For this review, take the finished solid that the model builds, in its own axes (mm). A direction names the side the tool comes from. Give positions to 0.01 mm unless a question says otherwise; leave off trailing zeros. Order: outer loops, then holes, each group sorted by start corner. A loop starts at its lowest first (then second) coordinate and runs counter-clockwise, first axis right, second up.
from build123d import *

# Parameters (mm, degrees)
BOSS_EXTRUDE1_DEPTH = 110
CUT_EXTRUDE1_DEPTH  = 109
SKETCH3_R           = 2.875
CUT_EXTRUDE2_DEPTH  = 5


with BuildPart() as part:
    # Sketch1 → Boss-Extrude1 (new body)
    with BuildSketch(Plane(origin=(0, 0, 0), x_dir=(1, 0, 0), z_dir=(0, 1, 0))):
        with BuildLine():
            Line((-43.883093525, -1.707733813), (1.116906475, -1.707733813))
            Line((1.116906475, -1.707733813), (1.116906475, 18.292266187))
            ThreePointArc((1.116906475, 18.292266187), (-21.383093525, 40.792266187), (-43.883093525, 18.292266187))
            Line((-43.883093525, 18.292266187), (-43.883093525, -1.707733813))
        make_face()
    extrude(amount=BOSS_EXTRUDE1_DEPTH)

    # Sketch2 → Cut-Extrude1 (cut)
    with BuildSketch(Plane(origin=(0, 110, 0), x_dir=(1, 0, 0), z_dir=(0, 1, 0))):
        with BuildLine():
            Line((-42.883093525, 16.292266187), (-42.883093525, 13.292266187))
            Line((-42.883093525, 13.292266187), (-38.883093525, 13.292266187))
            Line((-38.883093525, 13.292266187), (-38.883093525, 11.292266187))
            Line((-38.883093525, 11.292266187), (-42.883093525, 11.292266187))
            Line((-42.883093525, 11.292266187), (-42.883093525, -0.707733813))
            Line((-42.883093525, -0.707733813), (0.116906475, -0.707733813))
            Line((0.116906475, -0.707733813), (0.116906475, 11.292266187))
            Line((0.116906475, 11.292266187), (-3.883093525, 11.292266187))
            Line((-3.883093525, 11.292266187), (-3.883093525, 13.292266187))
            Line((-3.883093525, 13.292266187), (0.116906475, 13.292266187))
            Line((0.116906475, 13.292266187), (0.116906475, 16.292266187))
            Line((0.116906475, 16.292266187), (-3.883093525, 16.292266187))
            Line((-3.883093525, 16.292266187), (-3.883093525, 18.292266187))
            Line((-3.883093525, 18.292266187), (0.116906475, 18.292266187))
            ThreePointArc((0.116906475, 18.292266187), (-21.383093525, 39.792266187), (-42.883093525, 18.292266187))
            Line((-42.883093525, 18.292266187), (-38.883093525, 18.292266187))
            Line((-38.883093525, 18.292266187), (-38.883093525, 16.292266187))
            Line((-38.883093525, 16.292266187), (-42.883093525, 16.292266187))
        make_face()
    extrude(amount=-CUT_EXTRUDE1_DEPTH, mode=Mode.SUBTRACT)

    # Sketch3 → Cut-Extrude2 (cut)
    with BuildSketch(Plane.ZY.offset(43.883093525)):
        with Locations((-4.958932854, 55)):
            Circle(SKETCH3_R)
    extrude(amount=-CUT_EXTRUDE2_DEPTH, mode=Mode.SUBTRACT)


solid = part.part
1) Clearance check with flat-ended pins moving along their axes: pin 1 (1.5 mm diameter, centred on x = -26, z = -30, fed in from +Y); pin 2 (12 mm diameter, centred on x = -26.5, z = -26, fed in from -Y); pin 3 (13 mm diameter, centred on x = -27.5, y = 57.5, fed in from -Z); pin 4 (3 mm diameter, centred on x = -1.5, y = 80.5, fed in from -Z). State where each tip first meets the part, or that it passes through.
Answer sheet:
pin 1: stops at y = 1
pin 2: stops at y = 0
pin 3: stops at z = -40.79
pin 4: stops at z = -31.27
2) To check wall thickness, follow line 1 (X direction, y = 88.5, z = -13.5); line 2 (Z direction, x = -2, y = 5); line 3 (X direction, y = 49, z = -17). State the ranges of each line that lie inside material, in increasing order.
Answer sheet:
line 1: x = -43.88 to -42.88, 0.12 to 1.12
line 2: z = -29.72 to -27.6, -18.29 to -16.29, -13.29 to -11.29, 0.71 to 1.71
line 3: x = -43.88 to -38.88, -3.88 to 1.12
3) Tool access review of faces 1 (the face through (-22, 54, 1.708)), 2 (the face through (0.117, 56, -5)): name each direction out of +Z, -Z, +X, -X, +Y, -Y from which nothing blocks a thin tool from reaching the whole face with its end or side.
Answer sheet:
face 1: +Z, +X, -X, +Y, -Y
face 2: +Y
4) Draft analysis for pull direction Z (two halves, no side actions). For faces 3 (the face through (-23, 110, 1)), 4 (the face through (-20.888, 54.23, -40.787)), 5 (the face through (-42.883, 56, -15)), state which applies: +Z half, -Z half, draft (parallel to the pull), parting line (faces both ways), or undercut.
Answer sheet:
face 3: draft
face 4: -Z half
face 5: undercut
5) We need section A-A on y = 55. Give the boundary of the cut face in (x, z).
Answer sheet:
outline: (-43.88, -18.29) arc R22.5 ccw to (1.12, -18.29) - (1.12, 1.71) - (-43.88, 1.71) - (-43.88, -2.08) - (-42.88, -2.08) - (-42.88, 0.71) - (0.12, 0.71) - (0.12, -11.29) - (-3.88, -11.29) - (-3.88, -13.29) - (0.12, -13.29) - (0.12, -16.29) - (-3.88, -16.29) - (-3.88, -18.29) - (0.12, -18.29) arc R21.5 cw to (-42.88, -18.29) - (-38.88, -18.29) - (-38.88, -16.29) - (-42.88, -16.29) - (-42.88, -13.29) - (-38.88, -13.29) - (-38.88, -11.29) - (-42.88, -11.29) - (-42.88, -7.83) - (-43.88, -7.83) - close
6) We need section D-D on x = -20. Give the boundary of the cut face in (y, z).
Answer sheet:
outline: (0, -40.75) - (110, -40.75) - (110, -39.75) - (1, -39.75) - (1, 0.71) - (110, 0.71) - (110, 1.71) - (0, 1.71) - close
7) We need section C-C on z = -4. Give the boundary of the cut face in (x, y), then the cut area to 3 significant figures.
Answer sheet:
outline: (-43.88, 0) - (1.12, 0) - (1.12, 110) - (0.12, 110) - (0.12, 1) - (-42.88, 1) - (-42.88, 52.29) - (-43.88, 52.29) - close; (-43.88, 57.71) - (-42.88, 57.71) - (-42.88, 110) - (-43.88, 110) - close
area: 258 mm2
8) We need section B-B on y = 18. Give the boundary of the cut face in (x, z), then the cut area to 3 significant figures.
Answer sheet:
outline: (-43.88, -18.29) arc R22.5 ccw to (1.12, -18.29) - (1.12, 1.71) - (-43.88, 1.71) - close; hole (-42.88, -18.29) arc R21.5 ccw to (0.12, -18.29) - (-3.88, -18.29) - (-3.88, -16.29) - (0.12, -16.29) - (0.12, -13.29) - (-3.88, -13.29) - (-3.88, -11.29) - (0.12, -11.29) - (0.12, 0.71) - (-42.88, 0.71) - (-42.88, -11.29) - (-38.88, -11.29) - (-38.88, -13.29) - (-42.88, -13.29) - (-42.88, -16.29) - (-38.88, -16.29) - (-38.88, -18.29) - close
area: 184 mm2
